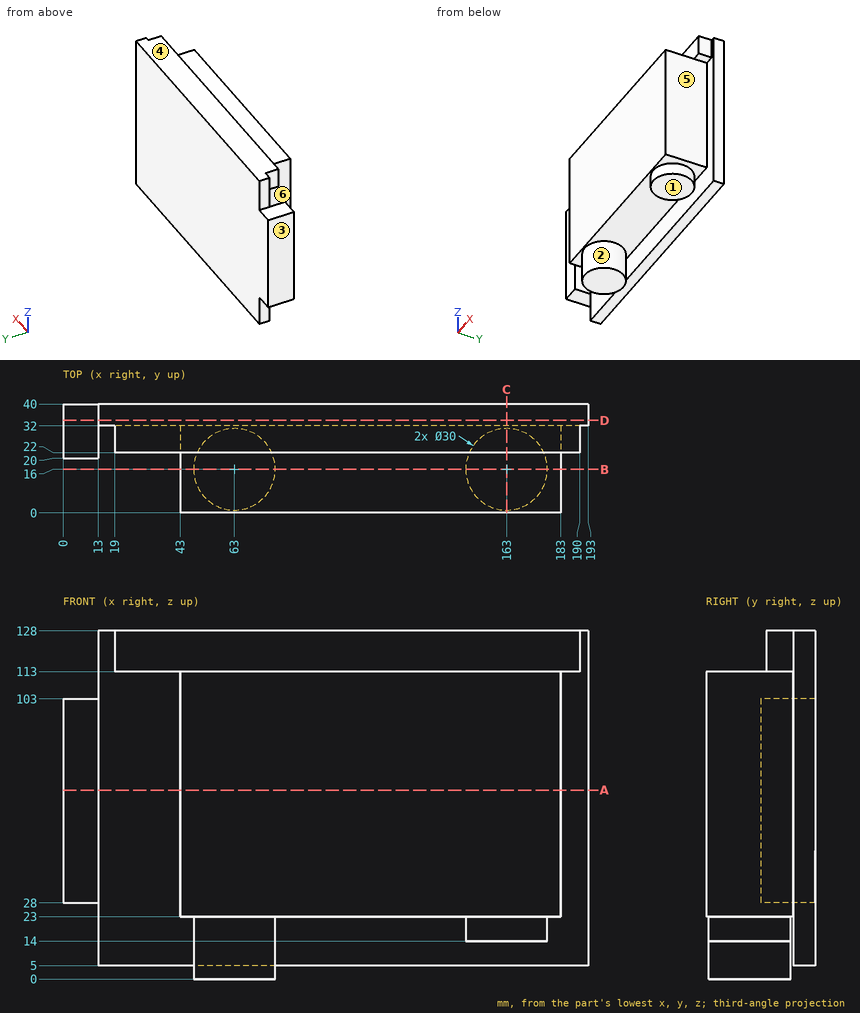
Can you work these out from the drawing? Everything is in mm from the part's minimum corner. A direction names the side the tool comes from. Give positions to 0.01 mm unless a question says otherwise; leave off trailing zeros. Loops run counter-clockwise (first coordinate to the right, second up) from the corner with the lowest first, then second, coordinate; pieces in that order, holes last. Notation, with made-up numbers: (70, -7.75) - (125, -7.75) arc R15 cw to (125, 5.25) - close; hole circle Ø9 at (30.5, 88.5). An arc over 180 degrees is marked (long way). Use one line per item in the form item = value.
1. I need wall thicknesses on probe 1 along X at (y, z) = (9, 112); probe 2 along Y at (x, z) = (81, 22); probe 3 along X at (y, z) = (24.5, 59). Which ranges of each line are inside material? Lowest first, please.
Response values:
probe_1 = 43 to 183
probe_2 = 32 to 40
probe_3 = 0 to 13, 43 to 183
2. I want a section at C-C (x = 163). Please give me the cut outline in (y, z), and give its area (3 significant figures).
Response values:
outline = (0, 23) - (1, 23) - (1, 14) - (31, 14) - (31, 23) - (32, 23) - (32, 5) - (40, 5) - (40, 128) - (22, 128) - (22, 113) - (0, 113) - close
area = 4,280 mm²
3. I want a section at B-B (y = 16). Please give me the cut outline in (x, z).
Response values:
outline = (43, 23) - (48, 23) - (48, 0) - (78, 0) - (78, 23) - (148, 23) - (148, 14) - (178, 14) - (178, 23) - (183, 23) - (183, 113) - (43, 113) - close
4. I want a section at A-A (z = 69.5). Please give me the cut outline in (x, y).
Response values:
outline = (0, 20) - (13, 20) - (13, 32) - (43, 32) - (43, 0) - (183, 0) - (183, 32) - (193, 32) - (193, 40) - (0, 40) - close
5. I'm going to push flat-ended pins straight in: pin 1 Ø11 at (y, z) = (26, 117) entering from +X; pin 2 Ø4.5 at (x, z) = (95.5, 117.5) entering from -Y; pin 3 Ø6.5 at (x, y) = (137, 15) entering from +Z. Where does each tip first touch, or does it pass through?
Response values:
pin_1 = 190
pin_2 = 22
pin_3 = 113
6. Thinking about a two-plate mould opening in X: for the marked faces 1, 2 and 3, which applies, released by +X, released by -X, zero draft, split by the parting line, or undercut?
Response values:
face_1 = zero draft
face_2 = undercut
face_3 = released by -X
7. On a 3-axis mill with a long thin cutter (end or side, diameter ignored), from which of +Z, -Z, +X, -X, +Y, -Y can I reach the whole of each face in a straight line? I mean the marked faces 4, 5 and 6. Say none if no direction works.
Response values:
face_4 = +Z, +X, -X, +Y, -Y
face_5 = -Z, +X, -Y
face_6 = -Z, -Y
8. I want a section at D-D (y = 34). Please give me the cut outline in (x, z), and give its area (3 significant figures).
Response values:
outline = (0, 28) - (13, 28) - (13, 5) - (193, 5) - (193, 128) - (13, 128) - (13, 103) - (0, 103) - close
area = 23,100 mm²
